Check sheet for the modelled part. Datum: model origin and axes. Units: mm. Face numbers are marked on the shaded views. Coordinates: 2 decimals unless noted, no trailing zeros. Write each loop counter-clockwise with the first axis right and the second up, starting at its lowest first coordinate (ties: lowest second). Pieces come first, ordered by that corner, then holes. Notation, with made-up numbers: (53.5, -9.75) - (80.5, -9.75) arc R7 ccw to (80.5, -0.75) - close; hole circle Ø5 at (75.5, 3.25). An arc over 180 degrees is marked (long way). Write each question's results on one line, items separated by ' | '.
from build123d import *

# Parameters (mm, degrees)
SKETCH1_W           = 40
SKETCH1_H           = 40
BOSS_EXTRUDE1_DEPTH = 3
SKETCH2_R           = 1
CUT_EXTRUDE1_DEPTH  = 10
SKETCH3_W           = 17
SKETCH3_H           = 17
CUT_EXTRUDE3_DEPTH  = 10
SKETCH4_W           = 2
SKETCH4_H           = 38
CUT_EXTRUDE4_DEPTH  = 41
CUT_EXTRUDE5_DEPTH  = 4


with BuildPart() as part:
    # Sketch1 → Boss-Extrude1 (new body)
    with BuildSketch(Plane.XY):
        with Locations((20, 20)):
            Rectangle(SKETCH1_W, SKETCH1_H)
    extrude(amount=BOSS_EXTRUDE1_DEPTH)

    # Sketch2 → Cut-Extrude1 (cut)
    with BuildSketch(Plane.XY.offset(3)):
        with Locations((3, 37)):
            Circle(SKETCH2_R)
        with Locations((3, 3)):
            Circle(SKETCH2_R)
        with Locations((37, 37)):
            Circle(SKETCH2_R)
        with Locations((37, 3)):
            Circle(SKETCH2_R)
    extrude(amount=-CUT_EXTRUDE1_DEPTH, mode=Mode.SUBTRACT)

    # Sketch3 → Cut-Extrude3 (cut)
    with BuildSketch(Plane(origin=(0, 0, 0), x_dir=(-1, 0, 0), z_dir=(0, 0, -1))):
        with Locations((-20, 20)):
            Rectangle(SKETCH3_W, SKETCH3_H)
    extrude(amount=-CUT_EXTRUDE3_DEPTH, mode=Mode.SUBTRACT)

    # Sketch4 → Cut-Extrude4 (cut, through all)
    with BuildSketch(Plane(origin=(40, 0, 0), x_dir=(0, 0, -1), z_dir=(1, 0, 0))):
        with Locations((-1, 20.024894978)):
            Rectangle(SKETCH4_W, SKETCH4_H)
    extrude(amount=-CUT_EXTRUDE4_DEPTH, mode=Mode.SUBTRACT)

    # Sketch7 → Cut-Extrude5 (cut, through all)
    with BuildSketch(Plane.XY.offset(3)):
        with BuildLine():
            Line((11.5, 22), (9.66485435, 22))
            ThreePointArc((9.66485435, 22), (7.66485435, 20), (9.66485435, 18))
            Line((9.66485435, 18), (11.5, 18))
            Line((11.5, 18), (11.5, 22))
        make_face()
        with BuildLine():
            Line((28.5, 22), (30.33514565, 22))
            ThreePointArc((30.33514565, 22), (32.33514565, 20), (30.33514565, 18))
            Line((30.33514565, 18), (28.5, 18))
            Line((28.5, 18), (28.5, 22))
        make_face()
    extrude(amount=-CUT_EXTRUDE5_DEPTH, mode=Mode.SUBTRACT)


solid = part.part
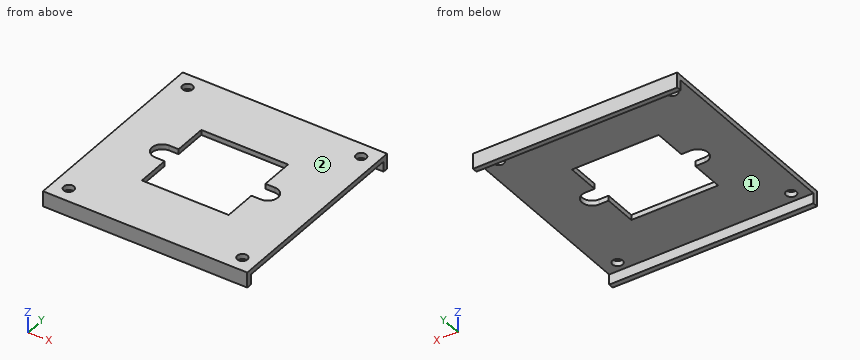
1. Sectioned sample at A-A (x = 28). Record the cut outline in (y, z).
Values follow:
outline: (0, 0) - (1.02, 0) - (1.02, 2) - (11.5, 2) - (11.5, 3) - (0, 3) - close; (28.5, 2) - (39.02, 2) - (39.02, 0) - (40, 0) - (40, 3) - (28.5, 3) - close
2. Sectioned sample at D-D (y = 37). Record the cut outline in (x, z).
Values follow:
outline: (0, 2) - (2, 2) - (2, 3) - (0, 3) - close; (4, 2) - (36, 2) - (36, 3) - (4, 3) - close; (38, 2) - (40, 2) - (40, 3) - (38, 3) - close
3. Sectioned sample at B-B (y = 14). Record the cut outline in (x, z), then the cut area to 3 significant figures.
Values follow:
outline: (0, 2) - (11.5, 2) - (11.5, 3) - (0, 3) - close; (28.5, 2) - (40, 2) - (40, 3) - (28.5, 3) - close | area: 23.0 mm^2
4. Sectioned sample at C-C (x = 3). Record the cut outline in (y, z), then the cut area to 3 significant figures.
Values follow:
outline: (0, 0) - (1.02, 0) - (1.02, 2) - (2, 2) - (2, 3) - (0, 3) - close; (4, 2) - (36, 2) - (36, 3) - (4, 3) - close; (38, 2) - (39.02, 2) - (39.02, 0) - (40, 0) - (40, 3) - (38, 3) - close | area: 40.0 mm^2
5. Draft check along Y on the marked faces 1 and 2. Enter one of: pulls with the +Y half, pulls with the -Y half, needs draft (parallel to the pull), parting line crosses it, or undercut.
Values follow:
face 1: undercut | face 2: needs draft
6. Go/stop test with flat-tipped pins: pin 1 (12 mm diameter, centred on x = 16, y = 17.5, fed in from -Z); pin 2 (1.8 mm diameter, centred on x = 37, y = 37, fed in from +Z). Record where each tip stops, or that it passes through.
Values follow:
pin 1: stops at z = 2 | pin 2: passes through
7. Material ranges on L1, parallel to Y at x = 3, z = 2.45; L2, parallel to Y at x = 33.5, z = 1.9; L3, parallel to Y at x = 24, z = 2.85, recorded low to high. Write a range as [from, to].
Values follow:
L1: y = [0, 2], [4, 36], [38, 40] | L2: y = [0, 1.02], [39.02, 40] | L3: y = [0, 11.5], [28.5, 40]
